```python
from build123d import *

# Parameters (mm, degrees)
F_8_1_8_1_DURCHMESSER_BOHRUNG1_D = 8.1
SKIZZE4_R                        = 1.55
SCHNITT_LINEAR_AUSTRAGEN1_DEPTH  = 47.652974182
FASE1_SIZE                       = 3.5
SKIZZE5_R                        = 1.55
SCHNITT_LINEAR_AUSTRAGEN2_DEPTH  = 47.652974182
FASE2_SIZE                       = 3.5


with BuildPart() as part:
    # Skizze1 → Rotation1 (revolve)
    with BuildSketch(Plane.XY, mode=Mode.PRIVATE) as rotation1_sk:
        Polygon((0, 0), (0, 16.5), (3, 16.5), (3, 32.5), (8, 32.5), (8, 0), align=None)
    revolve(rotation1_sk.sketch.rotate(Axis((0, 0, 0), (-1, 0, 0)), 90), axis=Axis((0, 0, 0), (-1, 0, 0)))

    # Ø8.1 (8.1) Durchmesser Bohrung1 (through all)
    with Locations(Plane.ZY):
        with Locations((0, 0)):
            Hole(F_8_1_8_1_DURCHMESSER_BOHRUNG1_D / 2)

    # Skizze4 → Schnitt-Linear austragen1 (cut, through all)
    with BuildSketch(Plane(origin=(8, 0, 0), x_dir=(0, 0, -1), z_dir=(1, 0, 0))):
        with Locations((0, 10)):
            Circle(SKIZZE4_R)
        with Locations((8.660254038, -5)):
            Circle(SKIZZE4_R)
        with Locations((-8.660254038, -5)):
            Circle(SKIZZE4_R)
    extrude(amount=-SCHNITT_LINEAR_AUSTRAGEN1_DEPTH, mode=Mode.SUBTRACT)

    # Fase1
    fase1_edges = [part.edges().sort_by_distance(p)[0] for p in [
        (8, 10, 1.55),
        (8, -5, -7.110254038),
        (8, -5, 10.210254038),
    ]]
    chamfer(fase1_edges, length=FASE1_SIZE)

    # Skizze5 → Schnitt-Linear austragen2 (cut, through all)
    with BuildSketch(Plane(origin=(8, 0, 0), x_dir=(0, 0, -1), z_dir=(1, 0, 0))):
        with Locations((0, 25)):
            Circle(SKIZZE5_R)
        with Locations((21.650635095, 12.5)):
            Circle(SKIZZE5_R)
        with Locations((21.650635095, -12.5)):
            Circle(SKIZZE5_R)
        with Locations((0, -25)):
            Circle(SKIZZE5_R)
        with Locations((-21.650635095, -12.5)):
            Circle(SKIZZE5_R)
        with Locations((-21.650635095, 12.5)):
            Circle(SKIZZE5_R)
    extrude(amount=-SCHNITT_LINEAR_AUSTRAGEN2_DEPTH, mode=Mode.SUBTRACT)

    # Fase2
    fase2_edges = [part.edges().sort_by_distance(p)[0] for p in [
        (3, 25, 1.55),
        (3, 12.5, 23.200635095),
        (3, -12.5, 23.200635095),
        (3, -25, 1.55),
        (3, -12.5, -20.100635095),
        (3, 12.5, -20.100635095),
    ]]
    chamfer(fase2_edges, length=FASE2_SIZE)


solid = part.part
```
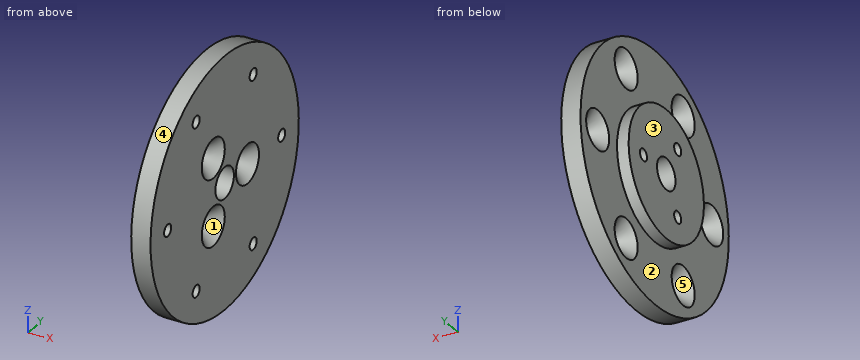
For this review, take the finished solid that the model builds, in its own axes (mm). Face numbers are marked on the shaded views. A direction names the side the tool comes from. Give positions to 0.01 mm unless a question says otherwise; leave off trailing zeros. Order: outer loops, then holes, each group sorted by start corner. A loop starts at its lowest first (then second) coordinate and runs counter-clockwise, first axis right, second up.
1) Take a section at B-B (y = -25). Give the boundary of the cut face in (x, z).
2) Take a section at A-A (z = 0). State how many separate pieces and enclosed holes the cut face has, then the cut area to 3 significant figures.
3) The part is to be moulded in two halves that separate along Y. For the marked faces 3, 4 and 5, say which applies: released by +Y, released by -Y, zero draft, split by the parting line, or undercut.
4) Wall thickness on line 1 (Y direction, x = 1.5, z = 0); line 2 (Z direction, x = 3.25, y = -14); line 3 (Y direction, x = 7.75, z = 3.5): over which ranges is each line inside the solid? List them lowest first.
5) Insertion check: pin 1 (3.5 mm diameter, centred on y = -5, z = -8.66, fed in from -X); pin 2 (3.5 mm diameter, centred on y = 25, z = 0, fed in from -X); pin 3 (4 mm diameter, centred on x = 7, z = 18, fed in from -Y); pin 4 (2 mm diameter, centred on x = 1.5, y = 23.5, fed in from -Z). Each pin has a flat end and moves straight along its axis. Give the tip position at first contact, or say it passes through.
6) For the marked faces 1 and 2, list the 3-axis set-ups (+Z, -Z, +X, -X, +Y, -Y) from which the entire face can be reached by the end or side of a thin tool; tool diameter is ignored.
7) Take a section at D-D (y = -5). Give the boundary of the cut face in (x, z), then the cut area to 3 significant figures.
Derived:
1. outline: (3, -20.77) - (8, -20.77) - (8, -1.55) - (6.5, -1.55) - (3, -5.05) - close; (3, 5.05) - (6.5, 1.55) - (8, 1.55) - (8, 20.77) - (3, 20.77) - close
2. separate pieces: 5
2. enclosed holes: 0
2. area: 267 mm2
3. face 3: zero draft
3. face 4: split by the parting line
3. face 5: undercut
4. line 1: y = -16.5 to -4.05, 4.05 to 8.45, 11.55 to 16.5
4. line 2: z = -29.33 to -26.21, -17.09 to 17.09, 26.21 to 29.33
4. line 3: y = -32.31 to -2.04, 2.04 to 6.72, 13.28 to 32.31
5. pin 1: stops at x = 0
5. pin 2: stops at x = 6.3
5. pin 3: stops at y = -28.29
5. pin 4: passes through
6. face 1: +X
6. face 2: -X
7. outline: (0, -15.72) - (3, -15.72) - (3, -32.11) - (8, -32.11) - (8, -13.71) - (4.5, -10.21) - (0, -10.21) - close; (0, -7.11) - (4.5, -7.11) - (8, -3.61) - (8, 3.61) - (4.5, 7.11) - (0, 7.11) - close; (0, 10.21) - (4.5, 10.21) - (8, 13.71) - (8, 32.11) - (3, 32.11) - (3, 15.72) - (0, 15.72) - close
7. area: 341 mm2
